Check sheet for the modelled part. Datum: model origin and axes. Units: mm. A direction names the side the tool comes from. Coordinates: 2 decimals unless noted, no trailing zeros. Write each loop counter-clockwise with the first axis right and the second up, starting at its lowest first coordinate (ties: lowest second). Pieces come first, ordered by that corner, then holes. Notation, with made-up numbers: (75, -28.75) -> (121, -28.75) arc R25 cw to (121, -4.75) -> close; hole circle Ø7 at (2, -23.75). An arc over 180 degrees is marked (long way). One line per item, written item: value. Start each with the question number.
1) Gauge pin test, flat ends, axial feed: P1, Ø10, axis at x = 824.5, z = -9.5, coming from the +Y side; P2, Ø6, axis at x = 801.34, y = 366.29, coming from the -Z side; P3, Ø1.5, axis at y = 335.5, z = -20.5, coming from the -X side; P4, Ø8, axis at x = 814, y = 335.5, coming from the -Z side. Record the tip position at first contact, or that the pin passes through.
2) Sectioned sample at A-A on z = -78.16. Enter the section's corners in (x, y).
3) Sectioned sample at B-B on x = 826. Enter the section's corners in (y, z), plus the area to 3 significant figures.
4) Set-up check for faces 4 (the flat face through (815, 322.351, 35)), 5 (the flat face through (797, 356.769, -9)), 6 (the flat face through (814.936, 364, -9)), 7 (the flat face through (800.966, 318, -18)): record each of +Z, -Z, +X, -X, +Y, -Y from which the full face is reachable in a straight line by a thin tool's end or side.
5) Scan lines: line 1 along Z through (x, y) = (798, 359.5); line 2 along Z through (x, y) = (822, 312); line 3 along X through (y, z) = (310.5, -78.5). Record each from-to range of solid material in increasing order. Write a range as [from, to].
6) Draft check along Y on faces 1 (the flat face through (815, 337, -31.75)), 2 (the flat face through (797, 352.959, -9)), 3 (the flat face through (804, 364, 0)). Enter one of: +Y half, -Y half, draft (parallel to the pull), parting line (faces both ways), or undercut.
7) Sectioned sample at D-D on y = 312. Enter the section's corners in (x, z) (3 decimals).
8) Sectioned sample at C-C on z = -13.5. Enter the section's corners in (x, y) (3 decimals), plus the area to 3 significant figures.
```python
from build123d import *

# Parameters (mm, degrees)
BOSS_EXTRUDE1_DEPTH = 21.59
SKETCH2_W           = 22.352
SKETCH2_H           = 21.6154
SKETCH2_R           = 3.2639
BOSS_EXTRUDE2_DEPTH = 3.81
BOSS_EXTRUDE3_START = -2.54
SKETCH3_R           = 3.2639
BOSS_EXTRUDE3_DEPTH = 2.54
SKETCH6_W           = 27.94
SKETCH6_H           = 142.24
SKETCH6_R           = 3.175
BOSS_EXTRUDE4_DEPTH = 48.388036719
SKETCH7_W           = 40.64
SKETCH7_H           = 30.608036719
SKETCH7_W_2         = 55.88
CUT_EXTRUDE1_DEPTH  = 30.226


with BuildPart() as part:
    # Sketch1 → Boss-Extrude1 (new body)
    with BuildSketch(Plane.XY):
        with BuildLine():
            Line((801.338321143, 356.769436719), (792.583825879, 356.769436719))
            Line((792.583825879, 356.769436719), (792.583825879, 352.959436719))
            Line((792.583825879, 352.959436719), (814.935825879, 352.959436719))
            Line((814.935825879, 352.959436719), (814.935825879, 374.574836719))
            Line((814.935825879, 374.574836719), (806.045825879, 374.574836719))
            ThreePointArc((806.045825879, 374.574836719), (810.863321143, 366.294436719), (806.045825879, 358.014036719))
            ThreePointArc((806.045825879, 358.014036719), (803.772947911, 357.085841957), (801.338321143, 356.769436719))
        make_face()
    extrude(amount=-BOSS_EXTRUDE1_DEPTH)

    # Sketch2 → Boss-Extrude2 (add)
    with BuildSketch(Plane.XY):
        with Locations((803.759825879, 363.767136719)):
            Rectangle(SKETCH2_W, SKETCH2_H)
        with Locations((801.338321143, 366.294436719)):
            Circle(SKETCH2_R, mode=Mode.SUBTRACT)
    extrude(amount=BOSS_EXTRUDE2_DEPTH)

    # Sketch3 → Boss-Extrude3 (add)
    with BuildSketch(Plane(origin=(0, 0, -21.59), x_dir=(-1, 0, 0), z_dir=(0, 0, -1)).offset(BOSS_EXTRUDE3_START)):
        with BuildLine():
            Line((-792.583825879, 356.769436719), (-792.583825879, 374.574836719))
            Line((-792.583825879, 374.574836719), (-806.045825879, 374.574836719))
            ThreePointArc((-806.045825879, 374.574836719), (-810.546915906, 363.859809951), (-801.338321143, 356.769436719))
            Line((-801.338321143, 356.769436719), (-792.583825879, 356.769436719))
        make_face()
        with Locations(Location((-801.338321143, 366.294436719, 0), (0, 0, 180))):
            Circle(SKETCH3_R, mode=Mode.SUBTRACT)
    extrude(amount=BOSS_EXTRUDE3_DEPTH)

    # Sketch6 → Boss-Extrude4 (add)
    with BuildSketch(Plane.XZ.offset(-352.959436719)):
        with Locations((814.935825879, -16.51)):
            Rectangle(SKETCH6_W, SKETCH6_H)
        with Locations(Location((820.039, 39.768571429, 0), (0, 0, 90))):
            Circle(SKETCH6_R, mode=Mode.SUBTRACT)
        with Locations(Location((820.039, -78.16, 0), (0, 0, 90))):
            Circle(SKETCH6_R, mode=Mode.SUBTRACT)
    extrude(amount=BOSS_EXTRUDE4_DEPTH)

    # Sketch7 → Cut-Extrude1 (cut)
    with BuildSketch(Plane(origin=(828.905825879, 0, 0), x_dir=(0, 0, -1), z_dir=(1, 0, 0))):
        with Locations((-34.29, 337.65541836)):
            Rectangle(SKETCH7_W, SKETCH7_H)
        with Locations((59.69, 337.65541836)):
            Rectangle(SKETCH7_W_2, SKETCH7_H)
    extrude(amount=-CUT_EXTRUDE1_DEPTH, mode=Mode.SUBTRACT)


solid = part.part
```
Answers:
1. P1: stops at y = 352.96
1. P2: passes through
1. P3: stops at x = 800.97
1. P4: stops at z = -31.75
2. outline: (800.97, 304.57) -> (816.86, 304.57) -> (816.86, 322.35) -> (800.97, 322.35) -> close; (823.21, 304.57) -> (828.91, 304.57) -> (828.91, 322.35) -> (823.21, 322.35) -> close
3. outline: (304.57, -87.63) -> (322.35, -87.63) -> (322.35, -31.75) -> (352.96, -31.75) -> (352.96, 13.97) -> (322.35, 13.97) -> (322.35, 54.61) -> (304.57, 54.61) -> close
3. area: 3,930 mm2
4. face 4: +Z, +X, -X, +Y
4. face 5: -X, +Y
4. face 6: +Z, -Z, +X, +Y
4. face 7: +Z, -Z, -X, -Y
5. line 1: z = [-21.59, -19.05], [0, 3.81]
5. line 2: z = [-87.63, -80.66], [-75.66, 37.27], [42.27, 54.61]
5. line 3: x = [800.97, 816.88], [823.2, 828.91]
6. face 1: draft
6. face 2: -Y half
6. face 3: undercut
7. outline: (800.966, -87.63) -> (828.906, -87.63) -> (828.906, 54.61) -> (800.966, 54.61) -> close; hole circle Ø6.35 at (820.039, -78.16); hole circle Ø6.35 at (820.039, 39.769)
8. outline: (792.584, 352.959) -> (800.966, 352.959) -> (800.966, 304.571) -> (828.906, 304.571) -> (828.906, 352.959) -> (814.936, 352.959) -> (814.936, 374.575) -> (806.046, 374.575) arc R9.525 cw to (801.338, 356.769) -> (792.584, 356.769) -> close
8. area: 1,540 mm2
